Can you work these out from the model? Positions are in its coordinate system, mm. Round coordinates to 2 decimals unless told otherwise and drop trailing zeros. Order: outer loops, then holes, each group sorted by start corner. A loop starts at its lowest first (then second) coordinate and runs counter-clockwise, first axis right, second up. Notation, with made-up numbers: (15, 15.5) -> (57, 15.5) arc R19 cw to (57, 32.5) -> close; hole circle Ø9 at (-12, 42). An arc over 180 degrees is marked (long way). One line per item, written item: value.
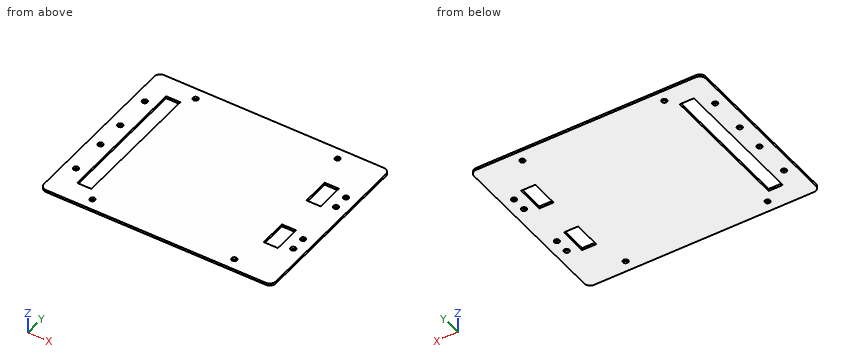
```python
from build123d import *

# Parameters (mm, degrees)
F0_R     = 1.75
F0_W     = 9.5
F0_H     = 90.5
F0_H_2   = 18.5
F1_DEPTH = 1.5


with BuildPart() as f1:
    # F0 (on Top) → F1 (new body)
    with BuildSketch(Plane.XY):
        with BuildLine():
            Line((73.5, 60), (-73.5, 60))
            ThreePointArc((-73.5, 60), (-76.328427, 58.828427), (-77.5, 56))
            Line((-77.5, 56), (-77.5, -56))
            ThreePointArc((-77.5, -56), (-76.328427, -58.828427), (-73.5, -60))
            Line((-73.5, -60), (73.5, -60))
            ThreePointArc((73.5, -60), (76.328427, -58.828427), (77.5, -56))
            Line((77.5, -56), (77.5, 56))
            ThreePointArc((77.5, 56), (76.328427, 58.828427), (73.5, 60))
        make_face()
        with Locations((-47.5, -52.5)):
            Circle(F0_R, mode=Mode.SUBTRACT)
        with Locations((-70, -35)):
            Circle(F0_R, mode=Mode.SUBTRACT)
        with Locations((-70, -10)):
            Circle(F0_R, mode=Mode.SUBTRACT)
        with Locations((-57.75, 0)):
            Rectangle(F0_W, F0_H, mode=Mode.SUBTRACT)
        with Locations((47.5, -52.5)):
            Circle(F0_R, mode=Mode.SUBTRACT)
        with Locations((57.75, -21.75)):
            Rectangle(F0_W, F0_H_2, mode=Mode.SUBTRACT)
        with Locations((70, -26.75)):
            Circle(F0_R, mode=Mode.SUBTRACT)
        with Locations((70, -16.75)):
            Circle(F0_R, mode=Mode.SUBTRACT)
        with Locations((-70, 10)):
            Circle(F0_R, mode=Mode.SUBTRACT)
        with Locations((-70, 35)):
            Circle(F0_R, mode=Mode.SUBTRACT)
        with Locations((-47.5, 52.5)):
            Circle(F0_R, mode=Mode.SUBTRACT)
        with Locations((57.75, 21.75)):
            Rectangle(F0_W, F0_H_2, mode=Mode.SUBTRACT)
        with Locations((70, 16.75)):
            Circle(F0_R, mode=Mode.SUBTRACT)
        with Locations((70, 26.75)):
            Circle(F0_R, mode=Mode.SUBTRACT)
        with Locations((47.5, 52.5)):
            Circle(F0_R, mode=Mode.SUBTRACT)
    extrude(amount=F1_DEPTH)


solid = f1.part
```
Q1. I want a section at C-C on z = 0.7. Give the number of separate pieces and of enclosed holes in the cut face, plus the area to 3 significant figures.
Answers below:
separate pieces: 1
enclosed holes: 15
area: 17,300 mm^2
Q2. I want a section at A-A on y = -16.75. List the corners of the cut face in (x, z) for me, plus the area to 3 significant figures.
Answers below:
outline: (-77.5, 0) -> (-62.5, 0) -> (-62.5, 1.5) -> (-77.5, 1.5) -> close; (-53, 0) -> (53, 0) -> (53, 1.5) -> (-53, 1.5) -> close; (62.5, 0) -> (68.25, 0) -> (68.25, 1.5) -> (62.5, 1.5) -> close; (71.75, 0) -> (77.5, 0) -> (77.5, 1.5) -> (71.75, 1.5) -> close
area: 199 mm^2
Q3. I want a section at B-B on x = -70. List the corners of the cut face in (y, z) for me, plus the area to 3 significant figures.
Answers below:
outline: (-60, 0) -> (-36.75, 0) -> (-36.75, 1.5) -> (-60, 1.5) -> close; (-33.25, 0) -> (-11.75, 0) -> (-11.75, 1.5) -> (-33.25, 1.5) -> close; (-8.25, 0) -> (8.25, 0) -> (8.25, 1.5) -> (-8.25, 1.5) -> close; (11.75, 0) -> (33.25, 0) -> (33.25, 1.5) -> (11.75, 1.5) -> close; (36.75, 0) -> (60, 0) -> (60, 1.5) -> (36.75, 1.5) -> close
area: 159 mm^2
Q4. I want a section at D-D on y = -35. List the corners of the cut face in (x, z) for me.
Answers below:
outline: (-77.5, 0) -> (-71.75, 0) -> (-71.75, 1.5) -> (-77.5, 1.5) -> close; (-68.25, 0) -> (-62.5, 0) -> (-62.5, 1.5) -> (-68.25, 1.5) -> close; (-53, 0) -> (77.5, 0) -> (77.5, 1.5) -> (-53, 1.5) -> close
Q5. Please list where these lines run through material, in increasing order: line 1 along X through (y, z) = (-19, 0.95); line 2 along Y through (x, z) = (-70, 0.7); line 3 along Y through (x, z) = (70, 0.4).
Answers below:
line 1: -77.5 to -62.5, -53 to 53, 62.5 to 77.5
line 2: -60 to -36.75, -33.25 to -11.75, -8.25 to 8.25, 11.75 to 33.25, 36.75 to 60
line 3: -60 to -28.5, -25 to -18.5, -15 to 15, 18.5 to 25, 28.5 to 60
